Geometry: final body of the model. Coordinates: model frame, mm. A direction names the side the tool comes from. Give positions to 0.01 mm unless a question says otherwise; leave off trailing zeros. Write each loop counter-clockwise with the first axis right and the second up, starting at its lowest first coordinate (ties: lowest second). Pieces come first, ordered by that corner, then holes.
Q1. Line query: L1, parallel to Y at x = 1.9, z = 0 (3 decimals); L2, parallel to Z at x = 97.5, y = 15; L3, parallel to X at y = 15.4, z = 17.5. Output: solid intervals per line, ascending.
Q2. Pin query (flat end, axial travel): pin 1 (2 mm diameter, centred on x = 97.5, z = -18.5, fed in from +Y) (3 decimals); pin 2 (1.6 mm diameter, centred on x = -8, y = -19, fed in from +Z); pin 3 (18.5 mm diameter, centred on y = 6.5, z = 5, fed in from -X); pin 4 (1.3 mm diameter, centred on y = -5.25, z = 0, fed in from +X). Return the tip coordinate at first contact, or that it passes through.
Q3. Reachability of faces 5 (the face through (38, 16.825, -23)), 6 (the face through (-9.9, -0.3, -26.9)), 7 (the face through (49, 0, -35)) from +Z, -Z, +X, -X, +Y, -Y: full face, straight path, thin tool, end or side. Return the list, or none.
Q4. Cut plane A-A on y = 0. Return the cut outline in (x, z), plus the area to 3 significant figures.
Q5. Cut plane C-C on z = -11.5. Return the cut outline in (x, y) (3 decimals).
Q6. Draft query along X for faces 1 (the face through (49, -2, 20)), 2 (the face through (100, 18, -24)), 3 (the face through (0, -1, -3)), 4 (the face through (0, 18, -24)). Return one class per face: pulls with the +X half, pulls with the -X half, needs draft (parallel to the pull), parting line crosses it, or undercut.
Q7. Cut plane D-D on y = -9.5. Return the cut outline in (x, z), plus the area to 3 significant figures.
```python
from build123d import *

# Parameters (mm, degrees)
BOSS_EXTRUDE1_DEPTH = 100
SHELL3_START        = 5
SHELL3_DEPTH        = 90
BOSS_EXTRUDE2_DEPTH = 20
SKETCH7_W           = 100
SKETCH7_H           = 50.81
CUT_EXTRUDE6_DEPTH  = 3.175
CUT_EXTRUDE1_REACH  = 130.062
SKETCH2_R           = 0.8
SKETCH2_R_2         = 3
SKETCH8_R           = 1
CUT_EXTRUDE7_DEPTH  = 3
CUT_EXTRUDE8_DEPTH  = 20
CUT_EXTRUDE9_START  = -20
CUT_EXTRUDE9_DEPTH  = 20


# Read off the part's stored shape, not the designer's step: Shell3
with BuildPart() as part:
    # Sketch1 → Boss-Extrude1 (new body)
    with BuildSketch(Plane(origin=(0, 0, 0), x_dir=(0, 0, -1), z_dir=(1, 0, 0))):
        with BuildLine():
            Line((-20, 20), (20, 20))
            ThreePointArc((20, 20), (40, 0), (20, -20))
            Line((20, -20), (-20, -20))
            Line((-20, -20), (-20, 20))
        make_face()
    extrude(amount=BOSS_EXTRUDE1_DEPTH)

    # Shell3 outline → Shell3 (cut)
    with BuildSketch(Plane.YZ.offset(SHELL3_START)):
        with BuildLine():
            Line((15, -20), (20, -20))
            Line((20, -20), (20, 15))
            Line((20, 15), (-15, 15))
            Line((-15, 15), (-15, -20))
            ThreePointArc((-15, -20), (0, -35), (15, -20))
        make_face()
    extrude(amount=SHELL3_DEPTH, mode=Mode.SUBTRACT)

    # Sketch9 → Boss-Extrude2 (add)
    with BuildSketch(Plane(origin=(100, 0, 0), x_dir=(0, 0, -1), z_dir=(1, 0, 0))):
        with BuildLine():
            Line((20, 20), (20, -20))
            ThreePointArc((20, -20), (40, 0), (20, 20))
        make_face()
    boss_extrude2 = extrude(amount=BOSS_EXTRUDE2_DEPTH)

    # Mirror1: Boss-Extrude2 across plane
    add(boss_extrude2.mirror(Plane(origin=(50, 0, 0), x_dir=(0, 0, 1), z_dir=(1, 0, 0))))

    # Sketch7 → Cut-Extrude6 (cut)
    with BuildSketch(Plane(origin=(0, 20, 0), x_dir=(1, 0, 0), z_dir=(0, 1, 0))):
        with Locations((50, 5.405)):
            Rectangle(SKETCH7_W, SKETCH7_H)
    extrude(amount=-CUT_EXTRUDE6_DEPTH, mode=Mode.SUBTRACT)

    # Cut-Extrude1: up to this face of the body (flat: up to its plane)
    cut_extrude1_end = Plane(part.part.faces().sort_by_distance((0, -1.5875, 0))[0])
    # Sketch2 → Cut-Extrude1 (cut, up to the picked face)
    with BuildSketch(Plane(origin=(100, 0, 0), x_dir=(0, 0, -1), z_dir=(1, 0, 0)), mode=Mode.PRIVATE) as cut_extrude1_sk1:
        with Locations(Location((0, -5.25, 0), (0, 0, 180))):
            Circle(SKETCH2_R)
    cut_extrude1_tool1 = split(extrude(cut_extrude1_sk1.sketch, amount=-CUT_EXTRUDE1_REACH, mode=Mode.PRIVATE), bisect_by=cut_extrude1_end, keep=Keep.BOTH, mode=Mode.PRIVATE)
    # Sketch2 → Cut-Extrude1 (cut, up to the picked face)
    with BuildSketch(Plane(origin=(100, 0, 0), x_dir=(0, 0, -1), z_dir=(1, 0, 0)), mode=Mode.PRIVATE) as cut_extrude1_sk2:
        with Locations(Location((0, 0, 0), (0, 0, 180))):
            Circle(SKETCH2_R_2)
    cut_extrude1_tool2 = split(extrude(cut_extrude1_sk2.sketch, amount=-CUT_EXTRUDE1_REACH, mode=Mode.PRIVATE), bisect_by=cut_extrude1_end, keep=Keep.BOTH, mode=Mode.PRIVATE)
    # Sketch2 → Cut-Extrude1 (cut, up to the picked face)
    with BuildSketch(Plane(origin=(100, 0, 0), x_dir=(0, 0, -1), z_dir=(1, 0, 0)), mode=Mode.PRIVATE) as cut_extrude1_sk3:
        with Locations(Location((0, 5.25, 0), (0, 0, 180))):
            Circle(SKETCH2_R)
    cut_extrude1_tool3 = split(extrude(cut_extrude1_sk3.sketch, amount=-CUT_EXTRUDE1_REACH, mode=Mode.PRIVATE), bisect_by=cut_extrude1_end, keep=Keep.BOTH, mode=Mode.PRIVATE)
    add(cut_extrude1_tool1.solids().sort_by(Axis((100, -5.25, 0), (-1, 0, 0)))[0], mode=Mode.SUBTRACT)
    add(cut_extrude1_tool2.solids().sort_by(Axis((100, 0, 0), (-1, 0, 0)))[0], mode=Mode.SUBTRACT)
    add(cut_extrude1_tool3.solids().sort_by(Axis((100, 5.25, 0), (-1, 0, 0)))[0], mode=Mode.SUBTRACT)

    # Sketch8 → Cut-Extrude7 (cut)
    with BuildSketch(Plane(origin=(0, 16.825, 0), x_dir=(1, 0, 0), z_dir=(0, 1, 0))):
        with Locations(Location((97.5, -17.5, 0), (0, 0, 270))):
            Circle(SKETCH8_R)
        with Locations(Location((97.5, 18.31, 0), (0, 0, 270))):
            Circle(SKETCH8_R)
        with Locations(Location((2.5, -17.5, 0), (0, 0, 90))):
            Circle(SKETCH8_R)
        with Locations(Location((2.5, 18.31, 0), (0, 0, 90))):
            Circle(SKETCH8_R)
    extrude(amount=-CUT_EXTRUDE7_DEPTH, mode=Mode.SUBTRACT)

    # Sketch10 → Cut-Extrude8 (cut)
    with BuildSketch(Plane(origin=(120, 0, 0), x_dir=(0, 0, -1), z_dir=(1, 0, 0))):
        with BuildLine():
            Line((20, 17.989163405), (20, -17.989163405))
            ThreePointArc((20, -17.989163405), (26.9, 0), (20, 17.989163405))
        make_face()
    extrude(amount=-CUT_EXTRUDE8_DEPTH, mode=Mode.SUBTRACT)

    # Sketch11 → Cut-Extrude9 (cut)
    with BuildSketch(Plane.ZY.offset(20).offset(CUT_EXTRUDE9_START)):
        with BuildLine():
            Line((-20, 17.989163405), (-20, -17.989163405))
            ThreePointArc((-20, -17.989163405), (-26.9, 0), (-20, 17.989163405))
        make_face()
    extrude(amount=CUT_EXTRUDE9_DEPTH, mode=Mode.SUBTRACT)


solid = part.part
```
Data:
1. L1: y = -20 to -6.05, -4.45 to -3, 3 to 4.45, 6.05 to 16.825
1. L2: z = -33.23 to -19.31, -17.31 to 16.5, 18.5 to 20
1. L3: x = 0 to 1.5, 3.5 to 96.5, 98.5 to 100
2. pin 1: stops at y = 16.825
2. pin 2: stops at z = -20
2. pin 3: stops at x = 0
2. pin 4: passes through
3. face 5: +Z, -Z, +Y
3. face 6: +Z, -X
3. face 7: none
4. outline: (-20, -40) - (120, -40) - (120, -26.9) - (100, -26.9) - (100, -3) - (95, -3) - (95, -35) - (5, -35) - (5, -3) - (0, -3) - (0, -26.9) - (-20, -26.9) - close; (0, 3) - (5, 3) - (5, 15) - (95, 15) - (95, 3) - (100, 3) - (100, 20) - (0, 20) - close
4. area: 1,960 mm2
5. outline: (0, -20) - (100, -20) - (100, 16.825) - (95, 16.825) - (95, -15) - (5, -15) - (5, 16.825) - (0, 16.825) - close
6. face 1: needs draft
6. face 2: undercut
6. face 3: pulls with the -X half
6. face 4: undercut
7. outline: (-20, -37.6) - (120, -37.6) - (120, -25.17) - (100, -25.17) - (100, 20) - (0, 20) - (0, -25.17) - (-20, -25.17) - close; hole (5, -31.61) - (95, -31.61) - (95, 15) - (5, 15) - close
7. area: 2,060 mm2
